Could you check a few things on this model? Use its own coordinates, in mm. A direction names the side the tool comes from. Give positions to 0.01 mm unless a question says otherwise; leave off trailing zeros. Order: outer loops, then holes, each group sorted by start corner. A loop starts at its lowest first (then second) coordinate and runs counter-clockwise, first axis right, second up. Notation, with made-up numbers: M -9.75,-20.75 L 34.25,-20.75 A31 cw 34.25,10.25 Z; hole C 58,79 d2. An arc over 180 degrees is marked long. Use a Markdown table: item, result. Add a question column.
```python
from build123d import *

# Parameters (mm, degrees)
BOSS_EXTRUDE1_DEPTH = 6
M3_TAPPED_HOLE1_D   = 2.5
FILLET1_R           = 3
FILLET2_R           = 0.5
FILLET3_R           = 0.25


with BuildPart() as part:
    # Sketch1 → Boss-Extrude1 (new body)
    with BuildSketch(Plane.XY):
        Polygon((3.1, 0), (-3.1, 0), (-3.1, -0.5), (-5, -0.5), (-5, -2), (-3, -4), (3, -4), (5, -2), (5, -0.5), (3.1, -0.5), align=None)
    extrude(amount=BOSS_EXTRUDE1_DEPTH)

    # M3 Tapped Hole1 (through all)
    with Locations(Plane(origin=(0, 0, 0), x_dir=(-1, 0, 0), z_dir=(0, 1, 0))):
        with Locations((0, 3)):
            Hole(M3_TAPPED_HOLE1_D / 2)

    # Fillet1
    fillet1_edges = [part.edges().sort_by_distance(p)[0] for p in [
        (-3.1, -0.25, 0),
        (3.1, -0.25, 6),
    ]]
    fillet(fillet1_edges, radius=FILLET1_R)

    # Fillet2
    fillet2_edges = [part.edges().sort_by_distance(p)[0] for p in [
        (5, -2, 3),
        (3, -4, 3),
        (-3, -4, 3),
        (-5, -2, 3),
    ]]
    fillet(fillet2_edges, radius=FILLET2_R)

    # Fillet3
    fillet3_edges = [part.edges().sort_by_distance(p)[0] for p in [
        (-5, -1.146446609, 6),
        (-5, -1.146446609, 0),
        (5, -1.146446609, 0),
        (5, -1.146446609, 6),
        (4, -3, 0),
        (0, -4, 0),
        (-4, -3, 0),
        (-2.984234935, -3.961939766, 0),
        (-4.961939766, -1.984234935, 0),
        (2.984234935, -3.961939766, 0),
        (4.961939766, -1.984234935, 0),
        (4, -3, 6),
        (-4, -3, 6),
        (0, -4, 6),
        (-2.984234935, -3.961939766, 6),
        (-4.961939766, -1.984234935, 6),
        (2.984234935, -3.961939766, 6),
        (4.961939766, -1.984234935, 6),
    ]]
    fillet(fillet3_edges, radius=FILLET3_R)


solid = part.part
```
1) Suppose I cut it at B-B on x = 0. Please give me the cut outline in (y, z), and give its area (3 significant figures).
2) Please list where these lines run through material, in increasing order: line 1 (Z direction, x = 0, y = -2.9); line 2 (Y direction, x = 3.25, z = 4.5); line 3 (X direction, y = -2.25, z = 1). Write a range as from..to.
3) We'd pull the mould along Z, two halves only. Please class faces 4 (the face through (3.96, -2.93, 5.93)), 5 (the face through (-3.93, -2.96, 0.07)), 6 (the face through (-0.16, -2.03, 4.24)), 7 (the face through (4, -0.5, 3)): pulls with the +Z half, pulls with the -Z half, needs draft (parallel to the pull), parting line crosses it, or undercut.
4) For pin 1 (2 mm diameter, centred on x = 0, z = 3, fed in from -Y); pin 2 (0.6 mm diameter, centred on y = 0, z = 4.5, fed in from -X); pin 3 (2 mm diameter, centred on x = -4, z = 0.5, fed in from +Y), each with a flat end and sliding along its axis, tell me the tip position at first contact or that it passes through.
5) For faces 1 (the face through (5, -1, 3)), 2 (the face through (2.24, -0.25, 5.1)), 3 (the face through (-4, -0.5, 2)), which set-ups out of +Z, -Z, +X, -X, +Y, -Y let a thin tool reach every point of the face, with its end or its side?
6) Suppose I cut it at D-D on x = -2. Please give me the cut outline in (y, z).
7) Suppose I cut it at C-C on x = 2.5. Please give me the cut outline in (y, z).
8) Suppose I cut it at A-A on y = -0.6. Please give me the cut outline in (x, z), and give its area (3 significant figures).
Values found:
| question | item | result |
|---|---|---|
| 1 | outline | M -4,0.25 A0.25 ccw -3.75,0 L 0,0 L 0,1.75 L -4,1.75 Z; M -4,4.25 L 0,4.25 L 0,6 L -3.75,6 A0.25 ccw -4,5.75 Z |
| 1 | area | 14.0 mm^2 |
| 2 | line 1 | z = 0..1.75, 4.25..6 |
| 2 | line 2 | y = -3.75..-0.5 |
| 2 | line 3 | x = -4.75..4.75 |
| 3 | face 4 | pulls with the +Z half |
| 3 | face 5 | pulls with the -Z half |
| 3 | face 6 | undercut |
| 3 | face 7 | needs draft |
| 4 | pin 1 | passes through |
| 4 | pin 2 | stops at x = -3.1 |
| 4 | pin 3 | stops at y = -0.5 |
| 5 | face 1 | +Z, -Z, +X, +Y, -Y |
| 5 | face 2 | +Z, +X, +Y |
| 5 | face 3 | -Z, -X, +Y |
| 6 | outline | M -4,0.25 A0.25 ccw -3.75,0 L -0.5,0 L -0.5,0.68 L 0,0.68 L 0,6 L -3.75,6 A0.25 ccw -4,5.75 Z |
| 7 | outline | M -4,0.25 A0.25 ccw -3.75,0 L 0,0 L 0,4.8 L -0.5,4.8 L -0.5,6 L -3.75,6 A0.25 ccw -4,5.75 Z |
| 8 | outline | M -5,0.25 A0.25 ccw -4.75,0 L 4.75,0 A0.25 ccw 5,0.25 L 5,5.75 A0.25 ccw 4.75,6 L -4.75,6 A0.25 ccw -5,5.75 Z; hole C 0,3 d2.5 |
| 8 | area | 55.0 mm^2 |
